from build123d import *

# Parameters (mm, degrees)
F1_DEPTH = 18
F2_R     = 5
F3_R     = 2.5


with BuildPart() as f1:
    # F0 (on Top) → F1 (new body)
    with BuildSketch(Plane.XY):
        with BuildLine():
            Line((0, 50), (0, 0))
            Line((0, 0), (100, 0))
            Line((100, 0), (100, 16))
            Line((100, 16), (53, 16))
            ThreePointArc((53, 16), (47.87868, 13.87868), (50, 19))
            Line((50, 19), (50, 31))
            ThreePointArc((50, 31), (47.87868, 36.12132), (53, 34))
            Line((53, 34), (100, 34))
            Line((100, 34), (100, 50))
            Line((100, 50), (0, 50))
        make_face()
    extrude(amount=F1_DEPTH)

    # F2
    f2_edges = [f1.edges().sort_by_distance(p)[0] for p in [
        (0, 0, 9),
        (0, 50, 9),
    ]]
    fillet(f2_edges, radius=F2_R)

    # F3
    f3_edges = [f1.edges().sort_by_distance(p)[0] for p in [
        (52.5, 0, 18),
        (52.5, 0, 0),
    ]]
    fillet(f3_edges, radius=F3_R)


solid = f1.part
Build history of the part. All positions in model axes, mm. A direction names the side the tool comes from. Round coordinates to 2 decimals unless told otherwise and drop trailing zeros. Write each loop counter-clockwise with the first axis right and the second up, starting at its lowest first coordinate (ties: lowest second). Pieces come first, ordered by that corner, then holes. Notation, with made-up numbers: M 26,82 L 57,82 A17 cw 57,91 Z; hole C -39.5,55.25 d2. An arc over 180 degrees is marked long. Answer in a Markdown table with one row per item.
1. Flat gauge pins, fed straight in: P1, Ø5, axis at x = 50, y = 34, coming from the +Z side; P2, Ø9.5, axis at y = 25, z = 13, coming from the +X side. Where does each tip first touch, or does it go through?
Geometry check:
| item | result |
|---|---|
| P1 | through |
| P2 | x = 50 |
2. Saw through at B-B (z = 13.5). List the corners of the cut face in (x, y), and give its area (3 significant figures).
Geometry check:
| item | result |
|---|---|
| outline | M 0,5 A5 ccw 5,0 L 100,0 L 100,16 L 53,16 A3 cw long 50,19 L 50,31 A3 cw long 53,34 L 100,34 L 100,50 L 5,50 A5 ccw 0,45 Z |
| area | 4,050 mm2 |
3. Mould opens along Y. For faces 1 (the face through (50, 25, 9)), 2 (the face through (0.752, 24.72, 0.713)), 3 (the face through (53, 50, 9)) say: +Y half, -Y half, draft (parallel to the pull), parting line (faces both ways), or undercut.
Geometry check:
| item | result |
|---|---|
| face 1 | undercut |
| face 2 | draft |
| face 3 | +Y half |
4. Which spindle directions (+Z, -Z, +X, -X, +Y, -Y) get a long thin tool onto all of the face, cutting with end or side? Do faces 4 (the face through (76, 34, 9)), 5 (the face through (47.81, 36.05, 8.87)). Say none if no direction does.
Geometry check:
| item | result |
|---|---|
| face 4 | +Z, -Z, +X |
| face 5 | +Z, -Z |
5. Saw through at C-C (y = 14). List the corners of the cut face in (x, z), and give its area (3 significant figures).
Geometry check:
| item | result |
|---|---|
| outline | M 0,2.5 A2.5 ccw 2.5,0 L 47.76,0 L 47.76,18 L 2.5,18 A2.5 ccw 0,15.5 Z; M 52.24,0 L 100,0 L 100,18 L 52.24,18 Z |
| area | 1,720 mm2 |
6. Saw through at D-D (x = 48). List the corners of the cut face in (y, z).
Geometry check:
| item | result |
|---|---|
| outline | M 0,2.5 A2.5 ccw 2.5,0 L 13.76,0 L 13.76,18 L 2.5,18 A2.5 ccw 0,15.5 Z; M 18.24,0 L 31.76,0 L 31.76,18 L 18.24,18 Z; M 36.24,0 L 47.5,0 A2.5 ccw 50,2.5 L 50,15.5 A2.5 ccw 47.5,18 L 36.24,18 Z |
7. Probe L1, parallel to Y at x = 68, z = 4.5; L2, parallel to X at y = 21, z = 11.25; L3, parallel to Y at x = 40.5, z = 1. List the from-to ranges inside material, lowest first. Write a range as [from, to].
Geometry check:
| item | result |
|---|---|
| L1 | [0, 16], [34, 50] |
| L2 | [0, 50] |
| L3 | [0.5, 49.5] |
8. Saw through at A-A (x = 93.5). List the corners of the cut face in (y, z).
Geometry check:
| item | result |
|---|---|
| outline | M 0,2.5 A2.5 ccw 2.5,0 L 16,0 L 16,18 L 2.5,18 A2.5 ccw 0,15.5 Z; M 34,0 L 47.5,0 A2.5 ccw 50,2.5 L 50,15.5 A2.5 ccw 47.5,18 L 34,18 Z |
